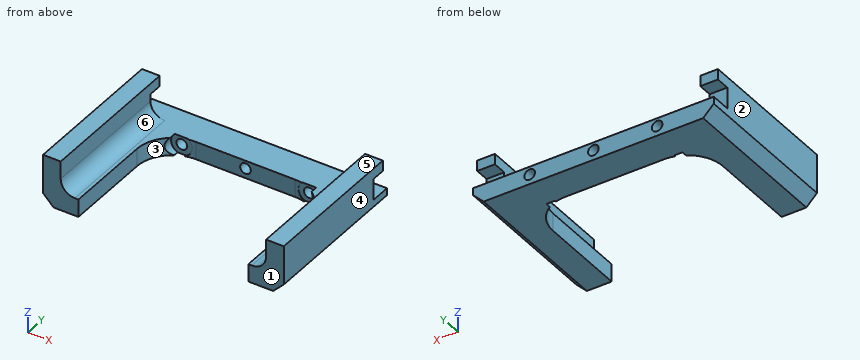
```python
from build123d import *

# Parameters (mm, degrees)
BOSS_EXTRUDE1_DEPTH     = 44
SKETCH2_W               = 48
SKETCH2_H               = 35
CUT_EXTRUDE1_DEPTH      = 15
FILLET1_R               = 10
SKETCH3_R               = 1.5
CUT_EXTRUDE2_DEPTH      = 36
CUT_EXTRUDE2_DEPTH_BACK = 10
CHAMFER1_SIZE           = 3
SKETCH4_W               = 9
SKETCH4_H               = 1.8
CUT_EXTRUDE3_DEPTH      = 35
CUT_EXTRUDE3_DEPTH_BACK = 35
SKETCH5_W               = 6
SKETCH5_H               = 3.971430967
CUT_EXTRUDE4_DEPTH      = 35
CUT_EXTRUDE4_DEPTH_BACK = 35
SKETCH6_R               = 3
CUT_EXTRUDE6_DEPTH      = 11
FILLET2_R               = 4


with BuildPart() as part:
    # Sketch1 → Boss-Extrude1 (new body)
    with BuildSketch(Plane(origin=(0, 0, 0), x_dir=(1, 0, 0), z_dir=(0, 1, 0))):
        Polygon((34, 0), (-34, 0), (-34, -14), (-29, -14), (-29, -5), (29, -5), (29, -14), (34, -14), align=None)
    extrude(amount=-BOSS_EXTRUDE1_DEPTH)

    # Sketch2 → Cut-Extrude1 (cut, through all)
    with BuildSketch(Plane(origin=(0, 0, 0), x_dir=(-1, 0, 0), z_dir=(0, 0, -1))):
        with Locations((0, -26.5)):
            Rectangle(SKETCH2_W, SKETCH2_H)
    extrude(amount=-CUT_EXTRUDE1_DEPTH, mode=Mode.SUBTRACT)

    # Fillet1
    fillet1_edges = [part.edges().sort_by_distance(p)[0] for p in [
        (-24, -9, 2.5),
        (24, -9, 2.5),
    ]]
    fillet(fillet1_edges, radius=FILLET1_R)

    # Sketch3 → Cut-Extrude2 (cut, two sides)
    with BuildSketch(Plane.XZ.offset(9)) as cut_extrude2_sk:
        with Locations((0, 2.75)):
            Circle(SKETCH3_R)
        with Locations((-18, 2.75)):
            Circle(SKETCH3_R)
        with Locations((18, 2.75)):
            Circle(SKETCH3_R)
    extrude(amount=CUT_EXTRUDE2_DEPTH, mode=Mode.SUBTRACT)
    extrude(cut_extrude2_sk.sketch, amount=-CUT_EXTRUDE2_DEPTH_BACK, mode=Mode.SUBTRACT)

    # Chamfer1
    chamfer1_edges = [part.edges().sort_by_distance(p)[0] for p in [
        (-34, -22, 0),
        (34, -22, 0),
    ]]
    chamfer(chamfer1_edges, length=CHAMFER1_SIZE)

    # Sketch4 → Cut-Extrude3 (cut, two sides)
    with BuildSketch(Plane(origin=(0, 0, 0), x_dir=(0, 0, -1), z_dir=(1, 0, 0))) as cut_extrude3_sk:
        with Locations((-9.5, -0.9)):
            Rectangle(SKETCH4_W, SKETCH4_H)
    extrude(amount=CUT_EXTRUDE3_DEPTH, mode=Mode.SUBTRACT)
    extrude(cut_extrude3_sk.sketch, amount=-CUT_EXTRUDE3_DEPTH_BACK, mode=Mode.SUBTRACT)

    # Sketch5 → Cut-Extrude4 (cut, two sides)
    with BuildSketch(Plane(origin=(0, 0, 0), x_dir=(0, 0, -1), z_dir=(1, 0, 0))) as cut_extrude4_sk:
        with Locations((-8, -3.785715484)):
            Rectangle(SKETCH5_W, SKETCH5_H)
    extrude(amount=CUT_EXTRUDE4_DEPTH, mode=Mode.SUBTRACT)
    extrude(cut_extrude4_sk.sketch, amount=-CUT_EXTRUDE4_DEPTH_BACK, mode=Mode.SUBTRACT)

    # Sketch6 → Cut-Extrude6 (cut)
    with BuildSketch(Plane.XZ.offset(9)):
        with Locations((0, 2.75)):
            Circle(SKETCH6_R)
        with Locations((18, 2.75)):
            Circle(SKETCH6_R)
        with Locations((-18, 2.75)):
            Circle(SKETCH6_R)
    extrude(amount=CUT_EXTRUDE6_DEPTH, mode=Mode.SUBTRACT)

    # Fillet2
    fillet2_edges = [part.edges().sort_by_distance(p)[0] for p in [
        (29, -24.885715483, 5),
        (-29, -24.885715483, 5),
    ]]
    fillet(fillet2_edges, radius=FILLET2_R)


solid = part.part
```
Can you work these out from the model? Positions are in its coordinate system, mm. Face numbers are marked on the shaded views. A direction names the side the tool comes from. Coordinates: 2 decimals unless noted, no trailing zeros. Order: outer loops, then holes, each group sorted by start corner. A loop starts at its lowest first (then second) coordinate and runs counter-clockwise, first axis right, second up.
1. If we section it at B-B (x = -18): Please give me the cut outline in (y, z), then the cut area to 3 significant figures.
2. If we section it at A-A (y = -3): Please give me the cut outline in (x, z), then the cut area to 3 significant figures.
3. If we section it at D-D (x = 8): Please give me the cut outline in (y, z).
4. If we section it at C-C (z = 6.25): Please give me the cut outline in (x, y), then the cut area to 3 significant figures.
5. Thinking about a two-plate mould opening in X: for the marked faces 1, 2, 3 and 4, which applies, +X half, -X half, draft (parallel to the pull), parting line (faces both ways), or undercut?
6. I need wall thicknesses on line 1 (X direction, y = -11, z = 10.5); line 2 (X direction, y = -6, z = 2); line 3 (Y direction, x = -20.5, z = 1.25). Which ranges of each line are inside material? Lowest first, please.
7. For the marked faces 5 and 6, which set-ups out of +Z, -Z, +X, -X, +Y, -Y let a thin tool reach every point of the face, with its end or its side?
8. I'm going to push flat-ended pins straight in: pin 1 (1.5 mm diameter, centred on y = -25.5, z = 1.5, fed in from +X); pin 2 (2 mm diameter, centred on x = -32.5, y = -4.5, fed in from -Z); pin 3 (3.5 mm diameter, centred on x = -32.5, z = 12.5, fed in from +Y). Where does each tip first touch, or does it pass through?
Entries:
1. outline: (-9, 0) - (0, 0) - (0, 1.25) - (-9, 1.25) - close; (-9, 4.25) - (0, 4.25) - (0, 5) - (-9, 5) - close
1. area: 18.0 mm2
2. outline: (-34, 3) - (-31, 0) - (31, 0) - (34, 3) - (34, 5) - (-34, 5) - close; (-34, 11) - (-29, 11) - (-29, 14) - (-34, 14) - close; (29, 11) - (34, 11) - (34, 14) - (29, 14) - close; hole circle Ø3 at (-18, 2.75); hole circle Ø3 at (0, 2.75); hole circle Ø3 at (18, 2.75)
2. area: 340 mm2
3. outline: (-9, 0) - (0, 0) - (0, 5) - (-9, 5) - close
4. outline: (-34, -44) - (-27.9, -44) - (-27.9, -5.77) - (-34, -5.77) - close; (27.9, -44) - (34, -44) - (34, -5.77) - (27.9, -5.77) - close
4. area: 466 mm2
5. face 1: draft
5. face 2: -X half
5. face 3: undercut
5. face 4: +X half
6. line 1: x = -34 to -29, 29 to 34
6. line 2: x = -33 to -19.3, -16.7 to -1.3, 1.3 to 16.7, 19.3 to 33
6. line 3: y = -9 to 0
7. face 5: +Z, +X, -X, +Y, -Y
7. face 6: +Z, +Y, -Y
8. pin 1: stops at x = 33.25
8. pin 2: stops at z = 0.5
8. pin 3: stops at y = -1.8
